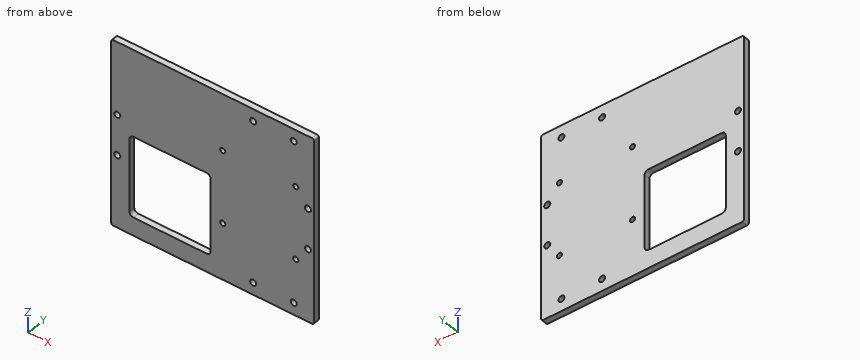
from build123d import *

# Parameters (mm, degrees)
SKETCH_1_W          = 100
SKETCH_1_H          = 92
EXTRUDE_1_DEPTH     = 3
SKETCH_2_R          = 1.5
CUT_EXTRUDE_1_DEPTH = 136.915414873
SKETCH_3_W          = 40
SKETCH_3_H          = 40
CUT_EXTRUDE_2_DEPTH = 10
FILLET_1_R          = 2
FILLET_2_R          = 1
SKETCH_4_R          = 1.25
CUT_EXTRUDE_3_DEPTH = 10


with BuildPart() as part:
    # 草图1 → 凸台-拉伸1 (new body)
    with BuildSketch(Plane(origin=(0, 0, 0), x_dir=(1, 0, 0), z_dir=(0, 1, 0))):
        with Locations((50, 46)):
            Rectangle(SKETCH_1_W, SKETCH_1_H)
    extrude(amount=EXTRUDE_1_DEPTH)

    # 草图2 → 切除-拉伸1 (cut, through all)
    with BuildSketch(Plane(origin=(0, 3, 0), x_dir=(1, 0, 0), z_dir=(0, 1, 0))):
        with Locations(Location((90, 86, 0), (0, 0, 270))):
            Circle(SKETCH_2_R)
        with Locations(Location((70, 86, 0), (0, 0, 270))):
            Circle(SKETCH_2_R)
        with Locations(Location((70, 6, 0), (0, 0, 270))):
            Circle(SKETCH_2_R)
        with Locations(Location((90, 6, 0), (0, 0, 270))):
            Circle(SKETCH_2_R)
        with Locations(Location((97, 56, 0), (0, 0, 270))):
            Circle(SKETCH_2_R)
        with Locations(Location((97, 36, 0), (0, 0, 270))):
            Circle(SKETCH_2_R)
        with Locations(Location((3, 36, 0), (0, 0, 90))):
            Circle(SKETCH_2_R)
        with Locations(Location((3, 56, 0), (0, 0, 90))):
            Circle(SKETCH_2_R)
    extrude(amount=-CUT_EXTRUDE_1_DEPTH, mode=Mode.SUBTRACT)

    # 草图3 → 切除-拉伸2 (cut)
    with BuildSketch(Plane(origin=(0, 3, 0), x_dir=(1, 0, 0), z_dir=(0, 1, 0))):
        with Locations((29, 63)):
            Rectangle(SKETCH_3_W, SKETCH_3_H)
    extrude(amount=-CUT_EXTRUDE_2_DEPTH, mode=Mode.SUBTRACT)

    # 圆角1
    fillet_1_edges = [part.edges().sort_by_distance(p)[0] for p in [
        (49, 1.5, -43),
        (9, 1.5, -43),
        (9, 1.5, -83),
        (49, 1.5, -83),
    ]]
    fillet(fillet_1_edges, radius=FILLET_1_R)

    # 圆角2
    fillet_2_edges = [part.edges().sort_by_distance(p)[0] for p in [
        (0, 1.5, -92),
        (100, 1.5, -92),
        (100, 1.5, 0),
        (0, 1.5, 0),
    ]]
    fillet(fillet_2_edges, radius=FILLET_2_R)

    # 草图4 → 切除-拉伸3 (cut)
    with BuildSketch(Plane.XZ):
        with Locations(Location((55, -28, 0), (0, 0, 270))):
            Circle(SKETCH_4_R)
        with Locations(Location((91, -28, 0), (0, 0, 270))):
            Circle(SKETCH_4_R)
        with Locations(Location((55, -64, 0), (0, 0, 270))):
            Circle(SKETCH_4_R)
        with Locations(Location((91, -64, 0), (0, 0, 270))):
            Circle(SKETCH_4_R)
    extrude(amount=-CUT_EXTRUDE_3_DEPTH, mode=Mode.SUBTRACT)


solid = part.part
Read the model definition and answer for the solid it produces. Units are mm, in the model's axes. Coordinates: 2 decimals unless noted, no trailing zeros. Loops run counter-clockwise (first coordinate to the right, second up) from the corner with the lowest first, then second, coordinate; pieces in that order, holes last. Notation, with made-up numbers: (20.5, 43.5) -> (57.5, 43.5) arc R16 ccw to (57.5, 74.5) -> close; hole circle Ø8 at (52.25, -39.75). An arc over 180 degrees is marked (long way). Write item = value, one per line. Start each with the question number.
1) Find the intervals of material crossed by L1, parallel to X at y = 1.6, z = -28; L2, parallel to X at y = 1.1, z = -6; L3, parallel to X at y = 0.7, z = -64, in increasing order. Write a range as from..to.
2) The part is cut by section B-B, the plane x = 29. Determine the outline of the cut face in (y, z).
3) The part is cut by section C-C, the plane z = -64. Determine the outline of the cut face in (x, y), plus the area to 3 significant figures.
4) The part is cut by section D-D, the plane y = 1.8. State how many separate pieces and enclosed holes the cut face has, plus the area to 3 significant figures.
5) Given P1, Ø2.5, axis at x = 97, z = -56, coming from the -Y side, flat-ended and moving along its own axis, determine where the tip first touches the part or whether it passes through.
6) The part is cut by section A-A, the plane z = -36. Determine the outline of the cut face in (x, y).
Result:
q1.L1 = 0..53.75, 56.25..89.75, 92.25..100
q1.L2 = 0..68.5, 71.5..88.5, 91.5..100
q1.L3 = 0..9, 49..53.75, 56.25..89.75, 92.25..100
q2.outline = (0, -92) -> (3, -92) -> (3, -83) -> (0, -83) -> close; (0, -43) -> (3, -43) -> (3, 0) -> (0, 0) -> close
q3.outline = (0, 0) -> (9, 0) -> (9, 3) -> (0, 3) -> close; (49, 0) -> (53.75, 0) -> (53.75, 3) -> (49, 3) -> close; (56.25, 0) -> (89.75, 0) -> (89.75, 3) -> (56.25, 3) -> close; (92.25, 0) -> (100, 0) -> (100, 3) -> (92.25, 3) -> close
q3.area = 165 mm²
q4.separate_pieces = 1
q4.enclosed_holes = 13
q4.area = 7,530 mm²
q5.P1 = through
q6.outline = (0, 0) -> (1.5, 0) -> (1.5, 3) -> (0, 3) -> close; (4.5, 0) -> (95.5, 0) -> (95.5, 3) -> (4.5, 3) -> close; (98.5, 0) -> (100, 0) -> (100, 3) -> (98.5, 3) -> close
